from build123d import *
from build123d import SkipClean  # not in build123d's __all__

# Parameters (mm, degrees)
F1_DEPTH = 10
F0_W     = 3
F0_H     = 7
F2_DEPTH = 40
F4_DEPTH = 48.42995
F5_R     = 1


# Not quite as in the source:
# - after a boolean that leaves OpenCascade's solid faulty, fix() repairs it


with BuildPart() as f1:
    # F0 (on Top) → F1 (new body)
    with BuildSketch(Plane.XY):
        with BuildLine():
            ThreePointArc((12.7, 16.05), (11.8213203436, 18.1713203436), (9.7, 19.05))
            Line((9.7, 19.05), (-9.7, 19.05))
            ThreePointArc((-9.7, 19.05), (-11.8213203436, 18.1713203436), (-12.7, 16.05))
            Line((-12.7, 16.05), (-12.7, 4.05))
            Line((-12.7, 4.05), (-9.7, 4.05))
            Line((-9.7, 4.05), (-9.7, -2.95))
            Line((-9.7, -2.95), (-12.7, -2.95))
            Line((-12.7, -2.95), (-12.7, -6.35))
            ThreePointArc((-12.7, -6.35), (-9.8244592727, -14.3979811133), (-2.5, -18.801505933))
            Line((-2.5, -18.801505933), (-2.5, -16.55))
            Line((-2.5, -16.55), (2.5, -16.55))
            Line((2.5, -16.55), (2.5, -18.801505933))
            ThreePointArc((2.5, -18.801505933), (9.8244592727, -14.3979811133), (12.7, -6.35))
            Line((12.7, -6.35), (12.7, -2.95))
            Line((12.7, -2.95), (9.7, -2.95))
            Line((9.7, -2.95), (9.7, 4.05))
            Line((9.7, 4.05), (12.7, 4.05))
            Line((12.7, 4.05), (12.7, 16.05))
        make_face()
    extrude(amount=F1_DEPTH)

    # F0 (on Top) → F2 (join)
    with BuildSketch(Plane.XY):
        with BuildLine():
            ThreePointArc((12.7, 16.05), (11.8213203436, 18.1713203436), (9.7, 19.05))
            Line((9.7, 19.05), (-9.7, 19.05))
            ThreePointArc((-9.7, 19.05), (-11.8213203436, 18.1713203436), (-12.7, 16.05))
            Line((-12.7, 16.05), (-12.7, 4.05))
            Line((-12.7, 4.05), (-9.7, 4.05))
            Line((-9.7, 4.05), (-9.7, -2.95))
            Line((-9.7, -2.95), (-12.7, -2.95))
            Line((-12.7, -2.95), (-12.7, -6.35))
            ThreePointArc((-12.7, -6.35), (-9.8244592727, -14.3979811133), (-2.5, -18.801505933))
            Line((-2.5, -18.801505933), (-2.5, -16.55))
            Line((-2.5, -16.55), (2.5, -16.55))
            Line((2.5, -16.55), (2.5, -18.801505933))
            ThreePointArc((2.5, -18.801505933), (9.8244592727, -14.3979811133), (12.7, -6.35))
            Line((12.7, -6.35), (12.7, -2.95))
            Line((12.7, -2.95), (9.7, -2.95))
            Line((9.7, -2.95), (9.7, 4.05))
            Line((9.7, 4.05), (12.7, 4.05))
            Line((12.7, 4.05), (12.7, 16.05))
        make_face()
        with Locations((11.2, 0.55)):
            Rectangle(F0_W, F0_H)
        with BuildLine():
            ThreePointArc((0, -19.05), (1.2561597531, -18.9877237933), (2.5, -18.801505933))
            Line((2.5, -18.801505933), (2.5, -16.55))
            Line((2.5, -16.55), (-2.5, -16.55))
            Line((-2.5, -16.55), (-2.5, -18.801505933))
            ThreePointArc((-2.5, -18.801505933), (-1.2561597531, -18.9877237933), (0, -19.05))
        make_face()
        with Locations((-11.2, 0.55)):
            Rectangle(F0_W, F0_H)
    with SkipClean():  # cleaning this boolean's faces spoils the solid; the shape is the same uncleaned
        extrude(amount=-F2_DEPTH)

    # F3 (on face) → F4 (cut)
    with BuildSketch(Plane(origin=(0, 0, -40), x_dir=(1, 0, 0), z_dir=(0, 0, -1))):
        with BuildLine():
            ThreePointArc((10.7, 6.35), (0, 17.05), (-10.7, 6.35))
            Line((-10.7, 6.35), (-10.7, -17.05))
            Line((-10.7, -17.05), (10.7, -17.05))
            Line((10.7, -17.05), (10.7, 6.35))
        make_face()
    extrude(amount=-F4_DEPTH, mode=Mode.SUBTRACT)

    add(f1.part.fix(), mode=Mode.REPLACE)

    # F5
    f5_edges = [f1.edges().sort_by_distance(p)[0] for p in [
        (9.824459, -14.397981, 10),
        (12.7, -4.65, 10),
        (11.2, -2.95, 10),
        (9.7, 0.55, 10),
        (11.2, 4.05, 10),
        (12.7, 10.05, 10),
        (11.82132, 18.17132, 10),
        (0, 19.05, 10),
        (-11.82132, 18.17132, 10),
        (-12.7, 10.05, 10),
        (-11.2, 4.05, 10),
        (-9.7, 0.55, 10),
        (-11.2, -2.95, 10),
        (-12.7, -4.65, 10),
        (-9.824459, -14.397981, 10),
        (-2.5, -17.675753, 10),
        (0, -16.55, 10),
        (2.5, -17.675753, 10),
    ]]
    fillet(f5_edges, radius=F5_R)


solid = f1.part
Could you check a few things on this model? Use its own coordinates, in mm. A direction names the side the tool comes from. Round coordinates to 2 decimals unless told otherwise and drop trailing zeros. Order: outer loops, then holes, each group sorted by start corner. A loop starts at its lowest first (then second) coordinate and runs counter-clockwise, first axis right, second up.
Q1. Imagine slicing it at D-D, the plane z = -28.5. List the corners of the cut face in (x, y) for me, then the cut area to 3 significant figures.
Geometry says:
outline: (-12.7, -6.35) arc R12.7 ccw to (12.7, -6.35) - (12.7, 16.05) arc R3 ccw to (9.7, 19.05) - (-9.7, 19.05) arc R3 ccw to (-12.7, 16.05) - close; hole (-10.7, -6.35) arc R10.7 ccw to (10.7, -6.35) - (10.7, 17.05) - (-10.7, 17.05) - close
area: 214 mm2
Q2. Thinking about a two-plate mould opening in X: for faces 1 (the face through (-12.7, 5, -15)), 2 (the face through (0, 1, 10)), 3 (the face through (2.5, -18, 4)), which applies, released by +X, released by -X, zero draft, split by the parting line, or undercut?
Geometry says:
face 1: released by -X
face 2: zero draft
face 3: undercut
Q3. Imagine slicing it at A-A, the plane y = 1. List the corners of the cut face in (x, z) for me, then the cut area to 3 significant figures.
Geometry says:
outline: (-12.7, -40) - (-10.7, -40) - (-10.7, 0) - (-12.7, 0) - close; (-9.7, 8.43) - (9.7, 8.43) - (9.7, 9) arc R1 ccw to (8.7, 10) - (-8.7, 10) arc R1 ccw to (-9.7, 9) - close; (10.7, -40) - (12.7, -40) - (12.7, 0) - (10.7, 0) - close
area: 190 mm2
Q4. Which directions (+Z, -Z, +X, -X, +Y, -Y) give clear straight access to the entire face, cutting with the end or side of a thin tool? Please do faces 4 (the face through (12, 4.05, 4)), 5 (the face through (0, -18, 0)), 6 (the face through (-12, 1, 0)), 7 (the face through (-12, -2.95, 4)).
Geometry says:
face 4: +Z, +X
face 5: +Z, -Y
face 6: +Z, +X, -X
face 7: +Z, -X
Q5. Please list where these lines run through material, in increasing order: probe 1 along X at (y, z) = (-1.5, -25); probe 2 along Z at (x, y) = (-6.75, -2); probe 3 along X at (y, z) = (17, -31.5).
Geometry says:
probe 1: x = -12.7 to -10.7, 10.7 to 12.7
probe 2: z = 8.43 to 10
probe 3: x = -12.55 to -10.7, 10.7 to 12.55
Q6. I'm going to push flat-ended pins straight in: P1, Ø1, axis at x = 11.5, y = 0.5, coming from the +Z side; P2, Ø1.1, axis at y = -17.5, z = 4.5, coming from the -X side (3 decimals); P3, Ø4, axis at x = 9, y = 3, coming from the +Z side; P4, Ø0.9, axis at x = 11, z = 3, coming from the +Y side. Where does each tip first touch, or does it pass through?
Geometry says:
P1: stops at z = 0
P2: stops at x = -6.995
P3: stops at z = 10
P4: stops at y = 18.93
Q7. Imagine slicing it at C-C, the plane x = -1.75. List the corners of the cut face in (y, z) for me.
Geometry says:
outline: (-18.93, -40) - (-16.91, -40) - (-16.91, 0) - (-18.93, 0) - close; (-16.55, 8.43) - (17.05, 8.43) - (17.05, -40) - (19.05, -40) - (19.05, 9) arc R1 ccw to (18.05, 10) - (-15.55, 10) arc R1 ccw to (-16.55, 9) - close
Q8. Imagine slicing it at B-B, the plane z = 2.5. List the corners of the cut face in (x, y) for me.
Geometry says:
outline: (-12.7, -6.35) arc R12.7 ccw to (-2.5, -18.8) - (-2.5, -16.75) arc R10.7 cw to (-10.7, -6.35) - (-10.7, -2.95) - (-12.7, -2.95) - close; (-12.7, 4.05) - (-10.7, 4.05) - (-10.7, 17.05) - (10.7, 17.05) - (10.7, 4.05) - (12.7, 4.05) - (12.7, 16.05) arc R3 ccw to (9.7, 19.05) - (-9.7, 19.05) arc R3 ccw to (-12.7, 16.05) - close; (2.5, -18.8) arc R12.7 ccw to (12.7, -6.35) - (12.7, -2.95) - (10.7, -2.95) - (10.7, -6.35) arc R10.7 cw to (2.5, -16.75) - close
